```python
from build123d import *

# Parameters (mm, degrees)
SKETCH1_W               = 65.0875
SKETCH1_H               = 36.5125
BOSS_EXTRUDE1_DEPTH     = 1.5875
SKETCH2_W               = 45.72
SKETCH2_H               = 2.38125
BOSS_EXTRUDE2_DEPTH     = 19.558
SKETCH3_W               = 1.016
SKETCH3_H               = 19.558
BOSS_EXTRUDE3_DEPTH     = 5.08
LPATTERN1_COUNT         = 10
LPATTERN1_PITCH         = 4.953
SKETCH4_R               = 6.35
BOSS_EXTRUDE4_DEPTH     = 19.05
SKETCH5_R               = 1.524
CUT_EXTRUDE1_DEPTH      = 19.05
MIRROR1_COPY_1_SKETCH_W = 1.016
MIRROR1_COPY_1_SKETCH_H = 19.558
MIRROR1_COPY_1_DEPTH    = 5.08
MIRROR1_COPY_2_SKETCH_W = 1.016
MIRROR1_COPY_2_SKETCH_H = 19.558
MIRROR1_COPY_2_DEPTH    = 5.08
MIRROR1_COPY_3_SKETCH_W = 1.016
MIRROR1_COPY_3_SKETCH_H = 19.558
MIRROR1_COPY_3_DEPTH    = 5.08
MIRROR1_COPY_4_SKETCH_W = 1.016
MIRROR1_COPY_4_SKETCH_H = 19.558
MIRROR1_COPY_4_DEPTH    = 5.08
MIRROR1_COPY_5_SKETCH_W = 1.016
MIRROR1_COPY_5_SKETCH_H = 19.558
MIRROR1_COPY_5_DEPTH    = 5.08
MIRROR1_COPY_6_SKETCH_W = 1.016
MIRROR1_COPY_6_SKETCH_H = 19.558
MIRROR1_COPY_6_DEPTH    = 5.08
MIRROR1_COPY_7_SKETCH_W = 1.016
MIRROR1_COPY_7_SKETCH_H = 19.558
MIRROR1_COPY_7_DEPTH    = 5.08
MIRROR1_COPY_8_SKETCH_W = 1.016
MIRROR1_COPY_8_SKETCH_H = 19.558
MIRROR1_COPY_8_DEPTH    = 5.08
MIRROR1_COPY_9_SKETCH_W = 1.016
MIRROR1_COPY_9_SKETCH_H = 19.558
MIRROR1_COPY_9_DEPTH    = 5.08
SKETCH6_R               = 11.43
SKETCH6_R_2             = 6.35
BOSS_EXTRUDE5_DEPTH     = 6.35
FILLET1_R               = 1.5875
SKETCH7_W               = 7.62
SKETCH7_H               = 19.812
BOSS_EXTRUDE6_DEPTH     = 10.16
CHAMFER1_SIZE           = 2.54
CHAMFER1_SIZE2          = 4.399409051
SKETCH8_W               = 4.7625
SKETCH8_H               = 9.525
BOSS_EXTRUDE7_DEPTH     = 10.31875


with BuildPart() as part:
    # Sketch1 → Boss-Extrude1 (new body)
    with BuildSketch(Plane(origin=(0, 0, 0), x_dir=(1, 0, 0), z_dir=(0, 1, 0))):
        Rectangle(SKETCH1_W, SKETCH1_H)
    extrude(amount=BOSS_EXTRUDE1_DEPTH)

    # Sketch2 → Boss-Extrude2 (add)
    with BuildSketch(Plane(origin=(0, 1.5875, 0), x_dir=(1, 0, 0), z_dir=(0, 1, 0))):
        with Locations((0, 15.478125)):
            Rectangle(SKETCH2_W, SKETCH2_H)
    boss_extrude2 = extrude(amount=BOSS_EXTRUDE2_DEPTH)

    # Sketch3 → Boss-Extrude3 (add)
    with BuildSketch(Plane(origin=(0, 0, -16.66875), x_dir=(-1, 0, 0), z_dir=(0, 0, -1))):
        with Locations((-22.352, 11.3665)):
            Rectangle(SKETCH3_W, SKETCH3_H)
    boss_extrude3 = extrude(amount=BOSS_EXTRUDE3_DEPTH)

    # LPattern1: Boss-Extrude3 ×10
    with Locations(*[(-i * LPATTERN1_PITCH, 0, 0) for i in range(1, LPATTERN1_COUNT)]):
        add(boss_extrude3)

    # Sketch4 → Boss-Extrude4 (add)
    with BuildSketch(Plane(origin=(0, 1.5875, 0), x_dir=(1, 0, 0), z_dir=(0, 1, 0))):
        with Locations(Location((13.335, 7.14375, 0), (0, 0, 90))):
            Circle(SKETCH4_R)
    boss_extrude4 = extrude(amount=BOSS_EXTRUDE4_DEPTH)

    # Sketch5 → Cut-Extrude1 (cut)
    with BuildSketch(Plane(origin=(0, 1.5875, 0), x_dir=(1, 0, 0), z_dir=(0, 1, 0))):
        with Locations(Location((29.49575, 13.68425, 0), (0, 0, 270))):
            Circle(SKETCH5_R)
        with Locations(Location((-29.384474521, 13.78665039, 0), (0, 0, 270))):
            Circle(SKETCH5_R)
    cut_extrude1 = extrude(amount=-CUT_EXTRUDE1_DEPTH, mode=Mode.SUBTRACT)

    # Mirror1: Boss-Extrude2, Boss-Extrude3, Boss-Extrude4, Cut-Extrude1 across plane
    add(boss_extrude2.mirror(Plane.XY))
    add(boss_extrude3.mirror(Plane.XY))
    add(boss_extrude4.mirror(Plane.XY))
    add(cut_extrude1.mirror(Plane.XY), mode=Mode.SUBTRACT)

    # Mirror1 copy 1 sketch → Mirror1 copy 1 (add)
    with BuildSketch(Plane(origin=(-4.953, 0, 16.66875), x_dir=(-1, 0, 0), z_dir=(0, 0, 1))):
        with Locations((-22.352, -11.3665)):
            Rectangle(MIRROR1_COPY_1_SKETCH_W, MIRROR1_COPY_1_SKETCH_H)
    extrude(amount=MIRROR1_COPY_1_DEPTH)

    # Mirror1 copy 2 sketch → Mirror1 copy 2 (add)
    with BuildSketch(Plane(origin=(-9.906, 0, 16.66875), x_dir=(-1, 0, 0), z_dir=(0, 0, 1))):
        with Locations((-22.352, -11.3665)):
            Rectangle(MIRROR1_COPY_2_SKETCH_W, MIRROR1_COPY_2_SKETCH_H)
    extrude(amount=MIRROR1_COPY_2_DEPTH)

    # Mirror1 copy 3 sketch → Mirror1 copy 3 (add)
    with BuildSketch(Plane(origin=(-14.859, 0, 16.66875), x_dir=(-1, 0, 0), z_dir=(0, 0, 1))):
        with Locations((-22.352, -11.3665)):
            Rectangle(MIRROR1_COPY_3_SKETCH_W, MIRROR1_COPY_3_SKETCH_H)
    extrude(amount=MIRROR1_COPY_3_DEPTH)

    # Mirror1 copy 4 sketch → Mirror1 copy 4 (add)
    with BuildSketch(Plane(origin=(-19.812, 0, 16.66875), x_dir=(-1, 0, 0), z_dir=(0, 0, 1))):
        with Locations((-22.352, -11.3665)):
            Rectangle(MIRROR1_COPY_4_SKETCH_W, MIRROR1_COPY_4_SKETCH_H)
    extrude(amount=MIRROR1_COPY_4_DEPTH)

    # Mirror1 copy 5 sketch → Mirror1 copy 5 (add)
    with BuildSketch(Plane(origin=(-24.765, 0, 16.66875), x_dir=(-1, 0, 0), z_dir=(0, 0, 1))):
        with Locations((-22.352, -11.3665)):
            Rectangle(MIRROR1_COPY_5_SKETCH_W, MIRROR1_COPY_5_SKETCH_H)
    extrude(amount=MIRROR1_COPY_5_DEPTH)

    # Mirror1 copy 6 sketch → Mirror1 copy 6 (add)
    with BuildSketch(Plane(origin=(-29.718, 0, 16.66875), x_dir=(-1, 0, 0), z_dir=(0, 0, 1))):
        with Locations((-22.352, -11.3665)):
            Rectangle(MIRROR1_COPY_6_SKETCH_W, MIRROR1_COPY_6_SKETCH_H)
    extrude(amount=MIRROR1_COPY_6_DEPTH)

    # Mirror1 copy 7 sketch → Mirror1 copy 7 (add)
    with BuildSketch(Plane(origin=(-34.671, 0, 16.66875), x_dir=(-1, 0, 0), z_dir=(0, 0, 1))):
        with Locations((-22.352, -11.3665)):
            Rectangle(MIRROR1_COPY_7_SKETCH_W, MIRROR1_COPY_7_SKETCH_H)
    extrude(amount=MIRROR1_COPY_7_DEPTH)

    # Mirror1 copy 8 sketch → Mirror1 copy 8 (add)
    with BuildSketch(Plane(origin=(-39.624, 0, 16.66875), x_dir=(-1, 0, 0), z_dir=(0, 0, 1))):
        with Locations((-22.352, -11.3665)):
            Rectangle(MIRROR1_COPY_8_SKETCH_W, MIRROR1_COPY_8_SKETCH_H)
    extrude(amount=MIRROR1_COPY_8_DEPTH)

    # Mirror1 copy 9 sketch → Mirror1 copy 9 (add)
    with BuildSketch(Plane(origin=(-44.577, 0, 16.66875), x_dir=(-1, 0, 0), z_dir=(0, 0, 1))):
        with Locations((-22.352, -11.3665)):
            Rectangle(MIRROR1_COPY_9_SKETCH_W, MIRROR1_COPY_9_SKETCH_H)
    extrude(amount=MIRROR1_COPY_9_DEPTH)

    # Sketch6 → Boss-Extrude5 (add)
    with BuildSketch(Plane(origin=(0, 1.5875, 0), x_dir=(1, 0, 0), z_dir=(0, 1, 0))):
        with Locations(Location((-14.76375, 0, 0), (0, 0, 270))):
            Circle(SKETCH6_R)
        with Locations(Location((-14.76375, 0, 0), (0, 0, 270))):
            Circle(SKETCH6_R_2, mode=Mode.SUBTRACT)
    extrude(amount=BOSS_EXTRUDE5_DEPTH)

    # Fillet1
    fillet1_edges = [part.edges().sort_by_distance(p)[0] for p in [
        (-14.76375, 7.9375, -11.43),
        (-14.76375, 7.9375, -6.35),
    ]]
    fillet(fillet1_edges, radius=FILLET1_R)

    # Sketch7 → Boss-Extrude6 (add)
    with BuildSketch(Plane(origin=(0, 1.5875, 0), x_dir=(1, 0, 0), z_dir=(0, 1, 0))):
        with Locations((27.94, 0)):
            Rectangle(SKETCH7_W, SKETCH7_H)
    extrude(amount=BOSS_EXTRUDE6_DEPTH)

    # Chamfer1
    chamfer1_edges = [part.edges().sort_by_distance(p)[0] for p in [
        (24.13, 11.7475, 0),
    ]]
    chamfer1_side = [part.faces().sort_by_distance(p)[0] for p in [
        (27.94, 11.7475, 0),
    ]]
    chamfer(chamfer1_edges, length=CHAMFER1_SIZE, length2=CHAMFER1_SIZE2, reference=chamfer1_side[0])

    # Sketch8 → Boss-Extrude7 (add)
    with BuildSketch(Plane(origin=(0, 1.5875, 0), x_dir=(1, 0, 0), z_dir=(0, 1, 0))):
        with Locations((-29.36875, 4.7625)):
            Rectangle(SKETCH8_W, SKETCH8_H)
    extrude(amount=BOSS_EXTRUDE7_DEPTH)


solid = part.part
```
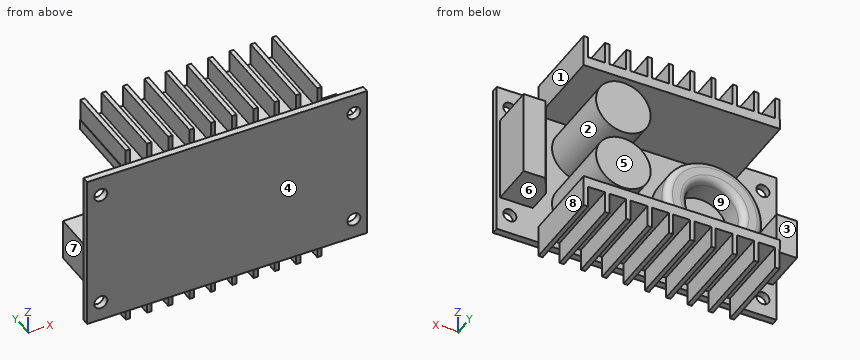
Part model, mm, in its own coordinate system. Face numbers are marked on the shaded views. A direction names the side the tool comes from. Coordinates: 2 decimals unless noted, no trailing zeros. Write item = value, one per line. Start each with the question number.
Item 1: Wall check: L1, parallel to Z at x = -17.5, y = 17.75; L2, parallel to Z at x = 20, y = 2.5; L3, parallel to Z at x = -16, y = 6.5. Give the ranges that are in metal, low to high. Write a range as from..to.
Item 2: Mould opens along X. For the marked faces 6, 7, 8 and 9 say: released by +X, released by -X, zero draft, split by the parting line, or undercut.
Item 3: Cut at A-A, the plane y = 9. State how many separate pieces and enclosed holes the cut face has, and give its area (3 significant figures).
Item 4: 3-axis set-ups, long thin cutter, end or side, ignore diameter. For the marked faces 1, 2, 3, 4 and 5: which of +Z, -Z, +X, -X, +Y, -Y reach the whole face in a straight line?
Item 5: Flat gauge pins, fed straight in: pin 1 Ø1.2 at (x, y) = (-10, 12.5) entering from -Z; pin 2 Ø2.5 at (y, z) = (6.5, 18.5) entering from +X; pin 3 Ø8 at (x, z) = (-7, 5.5) entering from +Y. Where does each tip first touch, or does it go through?
The answers:
q1.L1 = -21.75..-14.29, 14.29..21.75
q1.L2 = -16.67..-14.29, 14.29..16.67
q1.L3 = -16.67..-14.29, -11.36..-6.24, 6.24..11.36, 14.29..16.67
q2.face_6 = zero draft
q2.face_7 = released by -X
q2.face_8 = released by +X
q2.face_9 = undercut
q3.separate_pieces = 6
q3.enclosed_holes = 0
q3.area = 752 mm2
q4.face_1 = +Z, -Z, +X, +Y
q4.face_2 = +Y
q4.face_3 = +Z, -Z, -X, +Y
q4.face_4 = +Z, -Z, +X, -X, -Y
q4.face_5 = +X, -X, +Y
q5.pin_1 = -16.67
q5.pin_2 = 22.86
q5.pin_3 = 7.94
